```python
from build123d import *

# Parameters (mm, degrees)
SKETCH1_W               = 71.12
SKETCH1_H               = 106.68
BOSS_EXTRUDE1_DEPTH     = 87.884
SHELL1_T                = -10.16
SKETCH3_R               = 1.5875
CUT_EXTRUDE1_DEPTH      = 10.16
SKETCH4_W               = 81.28
SKETCH4_H               = 77.724
CUT_EXTRUDE2_DEPTH      = 72.12
CUT_EXTRUDE3_DEPTH      = 3.175
SKETCH7_W               = 45.72
SKETCH7_H               = 77.724
CUT_EXTRUDE4_DEPTH      = 1
CUT_EXTRUDE4_DEPTH_BACK = 107.68
SKETCH9_W               = 71.12
SKETCH9_H               = 106.68
CUT_EXTRUDE6_DEPTH      = 1.27
SKETCH10_R              = 14.986
SKETCH10_R_2            = 11.049
CUT_EXTRUDE7_DEPTH      = 7.112
SKETCH11_R              = 12.446
SKETCH11_R_2            = 8.509
CUT_EXTRUDE9_DEPTH      = 9.89
FILLET1_R               = 17.78


with BuildPart() as part:
    # Sketch1 → Boss-Extrude1 (new body)
    with BuildSketch(Plane(origin=(0, 0, 0), x_dir=(1, 0, 0), z_dir=(0, 1, 0))):
        with Locations((35.56, 53.34)):
            Rectangle(SKETCH1_W, SKETCH1_H)
    extrude(amount=BOSS_EXTRUDE1_DEPTH)

    # Shell1
    shell1_openings = [part.faces().sort_by_distance(p)[0] for p in [
        (35.56, 0, -53.34),
    ]]
    offset(amount=SHELL1_T, openings=shell1_openings, kind=Kind.INTERSECTION)

    # Sketch3 → Cut-Extrude1 (cut)
    with BuildSketch(Plane.XZ):
        with Locations((6.35, -6.35)):
            Circle(SKETCH3_R)
        with Locations((64.77, -6.35)):
            Circle(SKETCH3_R)
        with Locations((64.77, -100.33)):
            Circle(SKETCH3_R)
        with Locations((6.35, -100.33)):
            Circle(SKETCH3_R)
    extrude(amount=-CUT_EXTRUDE1_DEPTH, mode=Mode.SUBTRACT)

    # Sketch4 → Cut-Extrude2 (cut, through all)
    with BuildSketch(Plane.ZY):
        with Locations((-53.34, 38.862)):
            Rectangle(SKETCH4_W, SKETCH4_H)
    extrude(amount=-CUT_EXTRUDE2_DEPTH, mode=Mode.SUBTRACT)

    # Sketch6 → Cut-Extrude3 (cut)
    with BuildSketch(Plane.XZ):
        Polygon((69.536026472, -6.35), (67.153013236, -2.2225), (62.386986764, -2.2225), (60.003973528, -6.35), (62.386986764, -10.4775), (67.153013236, -10.4775), align=None)
        Polygon((11.116026472, -6.35), (8.733013236, -2.2225), (3.966986764, -2.2225), (1.583973528, -6.35), (3.966986764, -10.4775), (8.733013236, -10.4775), align=None)
        Polygon((69.536026472, -100.33), (67.153013236, -96.2025), (62.386986764, -96.2025), (60.003973528, -100.33), (62.386986764, -104.4575), (67.153013236, -104.4575), align=None)
        Polygon((11.116026472, -100.33), (8.733013236, -96.2025), (3.966986764, -96.2025), (1.583973528, -100.33), (3.966986764, -104.4575), (8.733013236, -104.4575), align=None)
    extrude(amount=-CUT_EXTRUDE3_DEPTH, mode=Mode.SUBTRACT)

    # Sketch7 → Cut-Extrude4 (cut, two sides)
    with BuildSketch(Plane(origin=(0, 0, -106.68), x_dir=(-1, 0, 0), z_dir=(0, 0, -1))) as cut_extrude4_sk:
        with Locations((-35.56, 38.862)):
            Rectangle(SKETCH7_W, SKETCH7_H)
    extrude(amount=CUT_EXTRUDE4_DEPTH, mode=Mode.SUBTRACT)
    extrude(cut_extrude4_sk.sketch, amount=-CUT_EXTRUDE4_DEPTH_BACK, mode=Mode.SUBTRACT)

    # Sketch9 → Cut-Extrude6 (cut)
    with BuildSketch(Plane(origin=(0, 87.884, 0), x_dir=(1, 0, 0), z_dir=(0, 1, 0))):
        with Locations((35.56, 53.34)):
            Rectangle(SKETCH9_W, SKETCH9_H)
    extrude(amount=-CUT_EXTRUDE6_DEPTH, mode=Mode.SUBTRACT)

    # Sketch10 → Cut-Extrude7 (cut)
    with BuildSketch(Plane(origin=(0, 77.724, 0), x_dir=(-1, 0, 0), z_dir=(0, -1, 0))):
        with Locations((-35.56, 27.94)):
            Circle(SKETCH10_R)
        with Locations((-35.56, 61.8744)):
            Circle(SKETCH10_R_2)
    extrude(amount=-CUT_EXTRUDE7_DEPTH, mode=Mode.SUBTRACT)

    # Sketch11 → Cut-Extrude9 (cut, through all)
    with BuildSketch(Plane.XZ.offset(-77.724)):
        with Locations((35.56, -27.94)):
            Circle(SKETCH11_R)
        with Locations((35.56, -61.8744)):
            Circle(SKETCH11_R_2)
    extrude(amount=-CUT_EXTRUDE9_DEPTH, mode=Mode.SUBTRACT)

    # Fillet1
    fillet1_edges = [part.edges().sort_by_distance(p)[0] for p in [
        (58.42, 77.724, -101.6),
        (58.42, 77.724, -5.08),
        (12.7, 77.724, -101.6),
        (12.7, 77.724, -5.08),
        (5.08, 77.724, -93.98),
        (5.08, 77.724, -12.7),
        (66.04, 77.724, -93.98),
        (66.04, 77.724, -12.7),
    ]]
    fillet(fillet1_edges, radius=FILLET1_R)


solid = part.part
```
Verification items for the finished model (mm, model axes). A direction names the side the tool comes from. Coordinates: 2 decimals unless noted, no trailing zeros. Loops run counter-clockwise (first coordinate to the right, second up) from the corner with the lowest first, then second, coordinate; pieces in that order, holes last. Notation, with made-up numbers: (10, 69.25) -> (34, 69.25) arc R9 cw to (34, 81.25) -> close; hole circle Ø8 at (62.25, 77). An arc over 180 degrees is marked (long way). Answer in a Markdown table with one row per item. Add a question column.
1. Draft check along X on faces 4 (the face through (5.15, 72.38, -17.77)), 5 (the face through (27, 77.724, -54)). Enter one of: +X half, -X half, draft (parallel to the pull), parting line (faces both ways), or undercut.
2. Material ranges on probe 1 along Z at (x, y) = (35.56, 85.4); probe 2 along Z at (x, y) = (35.56, 81); probe 3 along Z at (x, y) = (64.77, 8.75), recorded low to high. Write a range as [from, to].
3. Access from +Z, -Z, +X, -X, +Y, -Y to the whole of each face (thin tool, end or side, straight path). Record for faces 1 (the face through (12.7, 30, -5)), 2 (the face through (12, 47, -10.16)), 3 (the face through (5, 30, -93.98)).
4. Section check D-D, the plane x = 6.35. Enter the section's corners in (y, z) (1 decimal).
5. Section check C-C, the plane z = -27.94. Enter the section's corners in (x, y), then the cut area to 3 significant figures.
6. Depth check by flat-ended pin: P1, Ø6, axis at x = 45, z = -13, coming from the -Y side; P2, Ø2.5, axis at x = 65.5, z = -6, coming from the -Y side (3 decimals); P3, Ø13.5, axis at x = 35.56, z = -61.87, coming from the +Y side; P4, Ø8, axis at x = 54, z = -50, coming from the -Y side. Enter the tip coordinate at first touch or a pass-through.
7. Section check A-A, the plane x = 35.56. Enter the section's corners in (y, z), then the cut area to 3 significant figures.
8. Section check B-B, the plane y = 11.5. Enter the section's corners in (x, z).
Derived:
| question | item | result |
|---|---|---|
| 1 | face 4 | draft |
| 1 | face 5 | undercut |
| 2 | probe 1 | z = [-106.68, -70.38], [-53.37, -40.39], [-15.49, 0] |
| 2 | probe 2 | z = [-106.68, -72.92], [-50.83, -42.93], [-12.95, 0] |
| 2 | probe 3 | z = [-106.68, -101.92], [-98.74, -93.98], [-12.7, -7.94], [-4.76, 0] |
| 3 | face 1 | +Z, -Z, -Y |
| 3 | face 2 | -Y |
| 3 | face 3 | +X, -X, -Y |
| 4 | outline | (0, -106.7) -> (86.6, -106.7) -> (86.6, 0) -> (0, 0) -> (0, -2.2) -> (3.2, -2.2) -> (3.2, -4.8) -> (10.2, -4.8) -> (10.2, -7.9) -> (3.2, -7.9) -> (3.2, -10.5) -> (0, -10.5) -> (0, -12.7) -> (59.9, -12.7) arc R17.8 cw to (77.7, -30.5) -> (77.7, -76.2) arc R17.8 cw to (59.9, -94) -> (0, -94) -> (0, -96.2) -> (3.2, -96.2) -> (3.2, -98.7) -> (10.2, -98.7) -> (10.2, -101.9) -> (3.2, -101.9) -> (3.2, -104.5) -> (0, -104.5) -> close |
| 5 | outline | (0, 77.54) -> (10.16, 77.54) -> (10.16, 77.72) -> (20.57, 77.72) -> (20.57, 84.84) -> (23.11, 84.84) -> (23.11, 86.61) -> (0, 86.61) -> close; (48.01, 84.84) -> (50.55, 84.84) -> (50.55, 77.72) -> (60.96, 77.72) -> (60.96, 77.54) -> (71.12, 77.54) -> (71.12, 86.61) -> (48.01, 86.61) -> close |
| 5 | area | 379 mm² |
| 6 | P1 | stops at y = 76.91 |
| 6 | P2 | stops at y = 3.175 |
| 6 | P3 | passes through |
| 6 | P4 | stops at y = 77.72 |
| 7 | outline | (77.72, -106.68) -> (86.61, -106.68) -> (86.61, -70.38) -> (84.84, -70.38) -> (84.84, -72.92) -> (77.72, -72.92) -> close; (77.72, -50.83) -> (84.84, -50.83) -> (84.84, -53.37) -> (86.61, -53.37) -> (86.61, -40.39) -> (84.84, -40.39) -> (84.84, -42.93) -> (77.72, -42.93) -> close; (77.72, -12.95) -> (84.84, -12.95) -> (84.84, -15.49) -> (86.61, -15.49) -> (86.61, 0) -> (77.72, 0) -> close |
| 7 | area | 504 mm² |
| 8 | outline | (0, -106.68) -> (12.7, -106.68) -> (12.7, -96.52) -> (10.16, -96.52) -> (10.16, -93.98) -> (0, -93.98) -> close; (0, -12.7) -> (10.16, -12.7) -> (10.16, -10.16) -> (12.7, -10.16) -> (12.7, 0) -> (0, 0) -> close; (58.42, -106.68) -> (71.12, -106.68) -> (71.12, -93.98) -> (60.96, -93.98) -> (60.96, -96.52) -> (58.42, -96.52) -> close; (58.42, -10.16) -> (60.96, -10.16) -> (60.96, -12.7) -> (71.12, -12.7) -> (71.12, 0) -> (58.42, 0) -> close |
